Geometry: final body of the model. Coordinates: model frame, mm. Coordinates: 2 decimals unless noted, no trailing zeros. Order: outer loops, then holes, each group sorted by start corner. A loop starts at its lowest first (then second) coordinate and runs counter-clockwise, first axis right, second up. Notation, with made-up numbers: (31, -31) -> (41, -31) arc R26 cw to (41, -10) -> close; hole circle Ø11 at (63, 15). An arc over 180 degrees is marked (long way). Use CSV: the item, a comma, the result in double quotes. Start each with the question number.
from build123d import *

# Parameters (mm, degrees)
F0_W      = 42
F0_H      = 42
F1_DEPTH  = 1633
F2_W      = 42
F2_H      = 92
F3_DEPTH  = 2195
F6_W      = 42
F6_H      = 42
F7_DEPTH  = 2195
F9_DEPTH  = 116
F10_W     = 200
F10_H     = 100
F10_R     = 6
F11_DEPTH = 4
F12_W     = 50
F12_H     = 50
F12_W_2   = 42
F12_H_2   = 42
F13_DEPTH = 1633
F14_R     = 7
F15_DEPTH = 125
F16_R     = 15
F16_R_2   = 7
F17_DEPTH = 5


# Not quite as in the source:
# - a feature names something its author has since deleted; it is built from what else it names


with BuildPart() as f1:
    # F0 (on Top) → F1 (new body)
    with BuildSketch(Plane.XY):
        Polygon((0, 4), (0, 0), (50, 0), (50, 50), (0, 50), (0, 46), align=None)
        with Locations((25, 25)):
            Rectangle(F0_W, F0_H, mode=Mode.SUBTRACT)
    extrude(amount=F1_DEPTH)


with BuildPart() as f3:
    # F2 (on face) → F3 (new body)
    with BuildSketch(Plane(origin=(0, 0, 0), x_dir=(0, -1, 0), z_dir=(-1, 0, 0))):
        Polygon((0, 0), (-50, 0), (-50, -4), (-50, -96), (-50, -100), (0, -100), align=None)
        with Locations((-25, -50)):
            Rectangle(F2_W, F2_H, mode=Mode.SUBTRACT)
    extrude(amount=-F3_DEPTH)

    # F5: F1 across plane
    add(f1.part.mirror(Plane.YZ.offset(1097.5)))


with BuildPart() as f1_1:
    add(f1.part)

    add(f3.part)  # F7 merges F3
    # F6 (on face) → F7 (join, through all)
    with BuildSketch(Plane(origin=(0, 0, 0), x_dir=(0, -1, 0), z_dir=(-1, 0, 0))):
        Polygon((-46, 1683), (-50, 1683), (-50, 1633), (0, 1633), (0, 1683), (-4, 1683), align=None)
        with Locations((-25, 1658)):
            Rectangle(F6_W, F6_H, mode=Mode.SUBTRACT)
    extrude(amount=-F7_DEPTH)

    # F8 (on face) → F9 (join)
    with BuildSketch(Plane.YZ.offset(2195)):
        Polygon((4, 550), (0, 550), (0, 500), (50, 500), (50, 550), (46, 550), (46, 504), (4, 504), align=None)
        Polygon((0, 1500), (0, 1450), (4, 1450), (4, 1496), (46, 1496), (46, 1450), (50, 1450), (50, 1500), align=None)
    extrude(amount=F9_DEPTH)

    # F10 (on face) → F11 (join)
    with BuildSketch(Plane.YZ.offset(2311)):
        with Locations((25, 1450)):
            Rectangle(F10_W, F10_H)
        with Locations((-50, 1450)):
            Circle(F10_R, mode=Mode.SUBTRACT)
        with Locations((100, 1450)):
            Circle(F10_R, mode=Mode.SUBTRACT)
        with Locations((25, 550)):
            Rectangle(F10_W, F10_H)
        with Locations((-50, 550)):
            Circle(F10_R, mode=Mode.SUBTRACT)
        with Locations((100, 550)):
            Circle(F10_R, mode=Mode.SUBTRACT)
    extrude(amount=F11_DEPTH)

    # F12 (on face) → F13 (join, through all)
    with BuildSketch(Plane.XY):
        with Locations((265, 25)):
            Rectangle(F12_W, F12_H)
        with Locations((265, 25)):
            Rectangle(F12_W_2, F12_H_2, mode=Mode.SUBTRACT)
    extrude(amount=F13_DEPTH)

    # F14 (on face) → F15 (cut)
    with BuildSketch(Plane(origin=(0, 0, -100), x_dir=(1, 0, 0), z_dir=(0, 0, -1))):
        with Locations((150, -25)):
            Circle(F14_R)
        with Locations((500, -25)):
            Circle(F14_R)
        with Locations((850, -25)):
            Circle(F14_R)
        with Locations((1200, -25)):
            Circle(F14_R)
        with Locations((1550, -25)):
            Circle(F14_R)
        with Locations((1900, -25)):
            Circle(F14_R)
        with Locations((2250, -25)):
            Circle(F14_R)
    extrude(amount=-F15_DEPTH, mode=Mode.SUBTRACT)

    # F16 (on face) → F17 (cut)
    with BuildSketch(Plane.XY):
        with Locations((500, 25)):
            Circle(F16_R)
        with Locations((500, 25)):
            Circle(F16_R_2, mode=Mode.SUBTRACT)
        with Locations((850, 25)):
            Circle(F16_R)
        with Locations((850, 25)):
            Circle(F16_R_2, mode=Mode.SUBTRACT)
        with Locations((1200, 25)):
            Circle(F16_R)
        with Locations((1200, 25)):
            Circle(F16_R_2, mode=Mode.SUBTRACT)
        with Locations((1550, 25)):
            Circle(F16_R)
        with Locations((1550, 25)):
            Circle(F16_R_2, mode=Mode.SUBTRACT)
        with Locations((1900, 25)):
            Circle(F16_R)
        with Locations((1900, 25)):
            Circle(F16_R_2, mode=Mode.SUBTRACT)
        with Locations((150, 25)):
            Circle(F16_R)
    extrude(amount=-F17_DEPTH, mode=Mode.SUBTRACT)


solid = f1_1.part
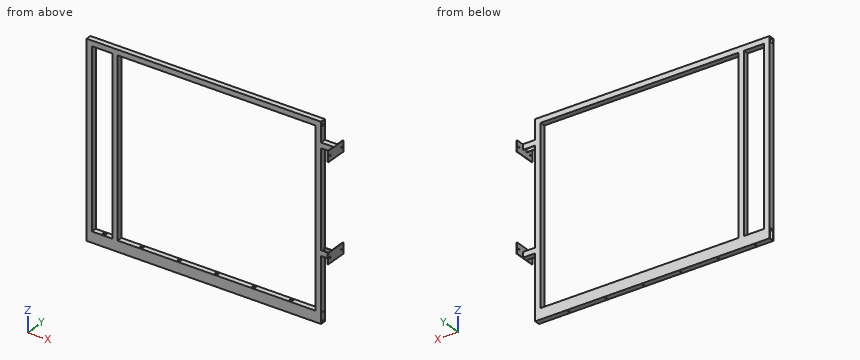
(1) Section B-B (z = 90.5). Return loops of the section in (x, y).
(2) First-contact query: pin 1 (4 mm diameter, centred on y = 0.5, z = 342, fed in from +X); pin 2 (11 mm diameter, centred on x = 150, y = 25, fed in from -Z); pin 3 (1.5 mm diameter, centred on x = 1552.5, y = -1, fed in from -Z). Flat tips, straight axial feed; report the tip coordinate or a pass-through.
(3) Line query: line 1 (Z direction, x = 1371.5, y = 10); line 2 (X direction, y = 12.5, z = 959); line 3 (Y direction, x = 500, z = -2). Output: solid intervals per line, ascending. Write a range as from..to.
(4) Section A-A (x = 912). Return loops of the section in (y, z).
Check sheet entries:
1,outline,"(0, 0) -> (50, 0) -> (50, 50) -> (0, 50) -> close; (240, 0) -> (290, 0) -> (290, 50) -> (240, 50) -> close; (2145, 0) -> (2195, 0) -> (2195, 50) -> (2145, 50) -> close; hole (4, 4) -> (46, 4) -> (46, 46) -> (4, 46) -> close; hole (244, 4) -> (286, 4) -> (286, 46) -> (244, 46) -> close; hole (2149, 4) -> (2191, 4) -> (2191, 46) -> (2149, 46) -> close"
2,pin 1,"stops at x = 2195"
2,pin 2,"stops at z = 1633"
2,pin 3,"passes through"
3,line 1,"z = -100..-96, -4..0, 1633..1637, 1679..1683"
3,line 2,"x = 0..4, 46..50, 240..244, 286..290, 2145..2149, 2191..2195"
3,line 3,"y = 0..10, 40..50"
4,outline,"(0, -100) -> (50, -100) -> (50, 0) -> (0, 0) -> close; (0, 1633) -> (50, 1633) -> (50, 1683) -> (0, 1683) -> close; hole (4, -96) -> (46, -96) -> (46, -4) -> (4, -4) -> close; hole (4, 1637) -> (46, 1637) -> (46, 1679) -> (4, 1679) -> close"
